Verification items for the finished model (mm, model axes). Face numbers are marked on the shaded views. A direction names the side the tool comes from. Coordinates: 2 decimals unless noted, no trailing zeros. Write each loop counter-clockwise with the first axis right and the second up, starting at its lowest first coordinate (ties: lowest second). Pieces come first, ordered by that corner, then holes. Notation, with made-up numbers: M 24.5,50 L 36.5,50 A28 cw 36.5,70 Z; hole C 39,36.5 d3. An arc over 180 degrees is marked long. One line per item, written item: value.
```python
from build123d import *

# Parameters (mm, degrees)
EXTRUDE_1_DEPTH      = 30
EXTRUDE_1_DEPTH_BACK = 30
SKETCH_1_W           = 150
SKETCH_1_H           = 100
FILLET_1_R           = 10
FILLET_2_R           = 10
SKETCH_2_R           = 25
EXTRUDE_2_DEPTH      = 25
SKETCH3_R            = 10
CUT_EXTRUDE1_DEPTH   = 137.788532191
SKETCH4_R            = 10
CUT_EXTRUDE2_DEPTH   = 125.384969617


with BuildPart() as part:
    # Sketch 1 → Extrude 1 (new, two sides: drawn at the far end of the back side and taken through both)
    with BuildSketch(Plane(origin=(0, 0, 0), x_dir=(1, 0, 0), z_dir=(0, 1, 0)).offset(-EXTRUDE_1_DEPTH_BACK)):
        with Locations((-0.40625, 0.6015625)):
            Rectangle(SKETCH_1_W, SKETCH_1_H)
    extrude(amount=EXTRUDE_1_DEPTH + EXTRUDE_1_DEPTH_BACK)

    # Fillet 1
    fillet_1_edges = [part.edges().sort_by_distance(p)[0] for p in [
        (-75.40625, 0, -50.6015625),
    ]]
    fillet(fillet_1_edges, radius=FILLET_1_R)

    # Fillet 2
    fillet_2_edges = [part.edges().sort_by_distance(p)[0] for p in [
        (74.59375, 0, -50.6015625),
        (74.59375, 0, 49.3984375),
        (-75.40625, 0, 49.3984375),
    ]]
    fillet(fillet_2_edges, radius=FILLET_2_R)

    # Sketch 2 → Extrude 2 (add)
    with BuildSketch(Plane(origin=(0, 30, 0), x_dir=(1, 0, 0), z_dir=(0, 1, 0))):
        with Locations(Location((0, 0, 0), (0, 0, 270))):
            Circle(SKETCH_2_R)
    extrude(amount=EXTRUDE_2_DEPTH)

    # Sketch3 → Cut-Extrude1 (cut, through all)
    with BuildSketch(Plane.XY.offset(49.3984375)):
        Circle(SKETCH3_R)
    extrude(amount=-CUT_EXTRUDE1_DEPTH, mode=Mode.SUBTRACT)

    # Sketch4 → Cut-Extrude2 (cut, through all)
    with BuildSketch(Plane(origin=(0, 55, 0), x_dir=(1, 0, 0), z_dir=(0, 1, 0))):
        with Locations(Location((-0.899046965, -4.468150991, 0), (0, 0, 270))):
            Circle(SKETCH4_R)
    extrude(amount=-CUT_EXTRUDE2_DEPTH, mode=Mode.SUBTRACT)


solid = part.part
```
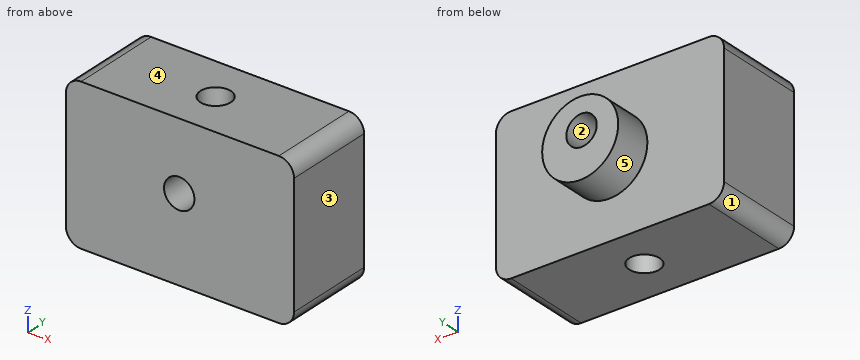
Item 1: Cross-section at C-C, the plane y = -23. Enter the section's corners in (x, z), and give its area (3 significant figures).
The answers:
outline: M -75.41,-40.6 A10 ccw -65.41,-50.6 L 64.59,-50.6 A10 ccw 74.59,-40.6 L 74.59,39.4 A10 ccw 64.59,49.4 L -65.41,49.4 A10 ccw -75.41,39.4 Z; hole C -0.9,4.47 d20
area: 14,600 mm²
Item 2: Cross-section at B-B, the plane y = 0. Enter the section's corners in (x, z).
The answers:
outline: M -75.41,-40.6 A10 ccw -65.41,-50.6 L -10,-50.6 L -10,0.32 A10 cw -10,8.61 L -10,49.4 L -65.41,49.4 A10 ccw -75.41,39.4 Z; M 10,-50.6 L 64.59,-50.6 A10 ccw 74.59,-40.6 L 74.59,39.4 A10 ccw 64.59,49.4 L 10,49.4 Z
Item 3: Access from +Z, -Z, +X, -X, +Y, -Y to the whole of each face (thin tool, end or side, straight path). Record for the marked faces 4 and 5.
The answers:
face 4: +Z, +X, -X, +Y, -Y
face 5: +Y
Item 4: Draft check along X on the marked faces 1, 2 and 3. Enter one of: released by +X, released by -X, zero draft, split by the parting line, or undercut.
The answers:
face 1: released by -X
face 2: undercut
face 3: released by +X
Item 5: Go/stop test with flat-tipped pins: P1, Ø10, axis at y = 41, z = -26.5, coming from the -X side; P2, Ø6, axis at x = 3, y = 45, coming from the +Z side; P3, Ø23, axis at x = 0, y = 0, coming from the -Z side; P4, Ø16, axis at x = -0.9, z = 4.47, coming from the +Y side. Record where each tip stops, or that it passes through.
The answers:
P1: stops at x = -12.76
P2: stops at z = 25
P3: stops at z = -50.6
P4: passes through
Item 6: Cross-section at A-A, the plane z = 29. Enter the section's corners in (x, y), and give its area (3 significant figures).
The answers:
outline: M -75.41,-30 L 74.59,-30 L 74.59,30 L -75.41,30 Z; hole C 0,0 d20
area: 8,690 mm²
Item 7: Cross-section at D-D, the plane x = 18. Enter the section's corners in (y, z).
The answers:
outline: M -30,-50.6 L 30,-50.6 L 30,-17.35 L 55,-17.35 L 55,17.35 L 30,17.35 L 30,49.4 L -30,49.4 Z
Item 8: Scan lines: line 1 (Y direction, x = 0, z = -13); line 2 (Y direction, x = 66.5, z = 45.5); line 3 (X direction, y = 0, z = 2). Record each from-to range of solid material in increasing order.
The answers:
line 1: y = -30 to -10, 10 to 55
line 2: y = -30 to 30
line 3: x = -75.41 to -10.59, 10 to 74.59
